Can you work these out from the drawing? Everything is in mm from the part's minimum corner. A direction names the side the tool comes from. Round coordinates to 2 decimals unless told otherwise and drop trailing zeros. Loops run counter-clockwise (first coordinate to the right, second up) from the corner with the lowest first, then second, coordinate; pieces in that order, holes last. Notation, with made-up numbers: (41.5, 6) - (81.5, 6) arc R16 cw to (81.5, 11) - close; hole circle Ø8 at (4, 62). An arc over 180 degrees is marked (long way). Return JSON: item names as keys, results as strings. Group by question number.
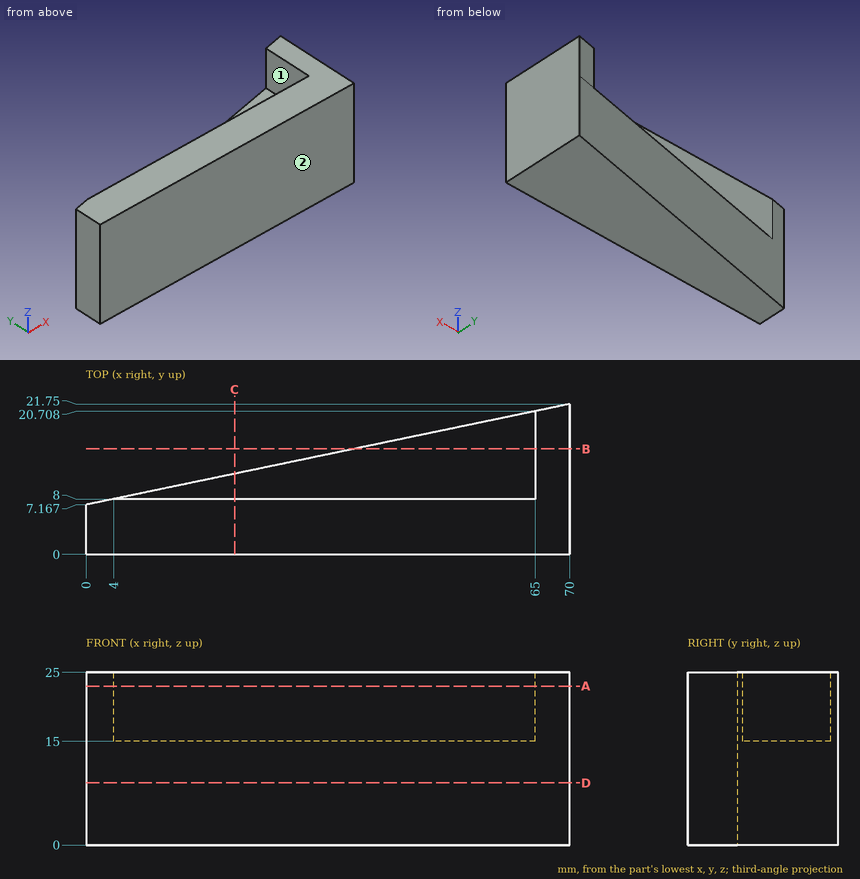
Q1. Imagine slicing it at D-D, the plane z = 9. List the corners of the cut face in (x, y) for me.
Q2. Imagine slicing it at B-B, the plane y = 15.25. List the corners of the cut face in (x, z) for me.
Q3. Will these pins go through, and if not, where does the flat tip stop? pin 1 Ø4 at (x, y) = (24, 16) entering from -Z; pin 2 Ø3 at (x, z) = (26.5, 18.5) entering from +Y; pin 3 Ø3 at (x, z) = (25.5, 9.5) entering from +Y; pin 4 Ø5 at (y, z) = (14, 22) entering from -X.
Q4. Please list where these lines run through material, in increasing order: line 1 (X direction, y = 16.25, z = 23.75); line 2 (Y direction, x = 51.5, z = 18.5); line 3 (Z direction, x = 26, y = 10).
Q5. Imagine slicing it at C-C, the plane x = 21.5. List the corners of the cut face in (y, z) for me.
Q6. For the marked faces 1 and 2, which set-ups out of +Z, -Z, +X, -X, +Y, -Y let a thin tool reach every point of the face, with its end or its side?
Q7. Imagine slicing it at A-A, the plane z = 23. List the corners of the cut face in (x, y) for me.
Output values:
{
 "1": {"outline": "(0, 0) - (70, 0) - (70, 21.75) - (0, 7.17) - close"},
 "2": {"outline": "(38.8, 0) - (70, 0) - (70, 25) - (65, 25) - (65, 15) - (38.8, 15) - close"},
 "3": {"pin 1": "passes through", "pin 2": "stops at y = 8", "pin 3": "stops at y = 12.79", "pin 4": "stops at x = 65"},
 "4": {"line 1": "x = 65 to 70", "line 2": "y = 0 to 8", "line 3": "z = 0 to 15"},
 "5": {"outline": "(0, 0) - (11.65, 0) - (11.65, 15) - (8, 15) - (8, 25) - (0, 25) - close"},
 "6": {"face 1": "+Z, -X, +Y", "face 2": "+Z, -Z, +X, -X, -Y"},
 "7": {"outline": "(0, 0) - (70, 0) - (70, 21.75) - (65, 20.71) - (65, 8) - (4, 8) - (0, 7.17) - close"}
}
